Build history of the part. All positions in model axes, mm. A direction names the side the tool comes from. Coordinates: 2 decimals unless noted, no trailing zeros. Loops run counter-clockwise (first coordinate to the right, second up) from the corner with the lowest first, then second, coordinate; pieces in that order, holes last.
Item 1: Mould opens along X. For faces 6 (the face through (94.38, 0.79, -65.22)), 7 (the face through (36.611, 0.789, -8.294)), 8 (the face through (56, 1.6, -36)), 9 (the face through (19.304, 0.789, -61.17)) say: released by +X, released by -X, zero draft, split by the parting line, or undercut.
Item 2: Cut at A-A (z = -32.5). List the corners of the cut face in (x, y), and give its area (3 significant figures).
Item 3: 3-axis set-ups, long thin cutter, end or side, ignore diameter. For faces 1 (the face through (17.121, 0.789, 0.224)), 2 (the face through (84.459, 0.789, 3.984)), 3 (the face through (79.23, 0.79, -50.7)), 4 (the face through (81.82, 0.79, -5.3)), 5 (the face through (88.41, 0.79, -71.1)): which of +Z, -Z, +X, -X, +Y, -Y reach the whole face in a straight line?
Item 4: Drill centre lines: line 1 along X through (y, z) = (1, -52.5); line 2 along X through (y, z) = (0.45, 0); line 3 along Z through (x, y) = (27.5, 0.75). Where is each one in solid material? Low to high.
Item 5: Cut at D-D (z = -49.5). List the corners of the cut face in (x, y), and give its area (3 significant figures).
Item 6: Flat gauge pin, fed straight in: pin 1 (0.5 mm diameter, centred on x = 58, y = 0.5, fed in from -Z). Where does the tip first touch, or does it go through?
Item 7: Cut at B-B (x = 59). List the corners of the cut face in (y, z), and give its area (3 significant figures).
Item 8: Cut at C-C (y = 0.95). Count the separate pieces of the cut face and the enclosed holes in it, and give its area (3 significant figures).
from build123d import *

# Parameters (mm, degrees)
EXTRUDE_1_DEPTH     = 1.6
SKETCH_2_R          = 3.5
SKETCH_2_R_2        = 1.5
CUT_EXTRUDE_2_DEPTH = 120.775748848


with BuildPart() as part:
    # 草图1 → 凸台-拉伸1 (new body)
    with BuildSketch(Plane(origin=(0, 0, 0), x_dir=(1, 0, 0), z_dir=(0, 1, 0))):
        with BuildLine():
            Line((47.950455462, 53.500678068), (63.550455462, 53.500678068))
            ThreePointArc((63.550455462, 53.500678068), (64.200939835, 53.197825288), (64.387892442, 52.505078257))
            ThreePointArc((64.387892442, 52.505078257), (64.672019835, 51.714227719), (65.496953127, 51.554046536))
            ThreePointArc((65.496953127, 51.554046536), (76.012452894, 57.657876981), (83.307978073, 67.384530764))
            ThreePointArc((83.307978073, 67.384530764), (84.439034072, 68.966777391), (86.050077403, 70.056424786))
            Line((86.050077403, 70.056424786), (90.83225012, 72.174467215))
            ThreePointArc((90.83225012, 72.174467215), (91.420402092, 72.243211116), (91.944318718, 71.967240399))
            Line((91.944318718, 71.967240399), (93.014982831, 70.896576286))
            Line((93.014982831, 70.896576286), (91.559408573, 69.441002029))
            ThreePointArc((91.559408573, 69.441002029), (92.166454693, 68.916677299), (92.690779423, 68.309631179))
            Line((92.690779423, 68.309631179), (94.146353681, 69.765205436))
            Line((94.146353681, 69.765205436), (95.217017793, 68.694541323))
            ThreePointArc((95.217017793, 68.694541323), (95.49298851, 68.170624698), (95.424244609, 67.582472725))
            Line((95.424244609, 67.582472725), (93.306202181, 62.800300009))
            ThreePointArc((93.306202181, 62.800300009), (92.216554786, 61.189256677), (90.634308158, 60.058200679))
            ThreePointArc((90.634308158, 60.058200679), (79.105768954, 50.532503354), (73.491163469, 36.671683358))
            ThreePointArc((73.491163469, 36.671683358), (73.672060349, 35.948096267), (74.303399444, 35.550965423))
            ThreePointArc((74.303399444, 35.550965423), (76.850455462, 32.500678068), (74.303399444, 29.450390712))
            ThreePointArc((74.303399444, 29.450390712), (73.672060349, 29.053259868), (73.491163469, 28.329672777))
            ThreePointArc((73.491163469, 28.329672777), (79.105768724, 14.468853095), (90.634307454, 4.94315579))
            ThreePointArc((90.634307454, 4.94315579), (92.216554514, 3.812099737), (93.306202181, 2.201056127))
            Line((93.306202181, 2.201056127), (95.424244609, -2.58111659))
            ThreePointArc((95.424244609, -2.58111659), (95.49298851, -3.169268563), (95.217017793, -3.693185188))
            Line((95.217017793, -3.693185188), (94.146353681, -4.763849301))
            Line((94.146353681, -4.763849301), (92.690779423, -3.308275044))
            ThreePointArc((92.690779423, -3.308275044), (92.166454693, -3.915321163), (91.559408573, -4.439645893))
            Line((91.559408573, -4.439645893), (93.014982831, -5.895220151))
            Line((93.014982831, -5.895220151), (91.944318718, -6.965884264))
            ThreePointArc((91.944318718, -6.965884264), (91.420402092, -7.24185498), (90.83225012, -7.173111079))
            Line((90.83225012, -7.173111079), (86.050077403, -5.055068651))
            ThreePointArc((86.050077403, -5.055068651), (84.439034072, -3.965421256), (83.307978073, -2.383174628))
            ThreePointArc((83.307978073, -2.383174628), (75.037180063, 8.17430315), (63.037239962, 14.163282556))
            ThreePointArc((63.037239962, 14.163282556), (61.901454693, 13.989537546), (61.221822682, 13.063094977))
            ThreePointArc((61.221822682, 13.063094977), (60.867876271, 12.514045024), (60.250455462, 12.300678068))
            Line((60.250455462, 12.300678068), (51.250455462, 12.300678068))
            ThreePointArc((51.250455462, 12.300678068), (50.633034654, 12.514045024), (50.279088243, 13.063094977))
            ThreePointArc((50.279088243, 13.063094977), (49.599456231, 13.989537546), (48.463670963, 14.163282556))
            ThreePointArc((48.463670963, 14.163282556), (36.463730861, 8.17430315), (28.192932851, -2.383174628))
            ThreePointArc((28.192932851, -2.383174628), (27.061876853, -3.965421256), (25.450833521, -5.055068651))
            Line((25.450833521, -5.055068651), (20.668660805, -7.173111079))
            ThreePointArc((20.668660805, -7.173111079), (20.080508832, -7.24185498), (19.556592206, -6.965884264))
            Line((19.556592206, -6.965884264), (18.485928094, -5.895220151))
            Line((18.485928094, -5.895220151), (19.941502351, -4.439645893))
            ThreePointArc((19.941502351, -4.439645893), (19.334456231, -3.915321163), (18.810131501, -3.308275044))
            Line((18.810131501, -3.308275044), (17.354557244, -4.763849301))
            Line((17.354557244, -4.763849301), (16.283893131, -3.693185188))
            ThreePointArc((16.283893131, -3.693185188), (16.007922414, -3.169268563), (16.076666315, -2.58111659))
            Line((16.076666315, -2.58111659), (18.194708744, 2.201056127))
            ThreePointArc((18.194708744, 2.201056127), (19.28435641, 3.812099737), (20.86660347, 4.94315579))
            ThreePointArc((20.86660347, 4.94315579), (32.395142201, 14.468853095), (38.009747455, 28.329672777))
            ThreePointArc((38.009747455, 28.329672777), (37.828850575, 29.053259868), (37.19751148, 29.450390712))
            ThreePointArc((37.19751148, 29.450390712), (34.650455462, 32.500678068), (37.19751148, 35.550965423))
            ThreePointArc((37.19751148, 35.550965423), (37.828850575, 35.948096267), (38.009747455, 36.671683358))
            ThreePointArc((38.009747455, 36.671683358), (32.39514197, 50.532503354), (20.866602766, 60.058200679))
            ThreePointArc((20.866602766, 60.058200679), (19.284356139, 61.189256677), (18.194708744, 62.800300009))
            Line((18.194708744, 62.800300009), (16.076666315, 67.582472725))
            ThreePointArc((16.076666315, 67.582472725), (16.007922414, 68.170624698), (16.283893131, 68.694541323))
            Line((16.283893131, 68.694541323), (17.354557244, 69.765205436))
            Line((17.354557244, 69.765205436), (18.810131501, 68.309631179))
            ThreePointArc((18.810131501, 68.309631179), (19.334456231, 68.916677299), (19.941502351, 69.441002029))
            Line((19.941502351, 69.441002029), (18.485928094, 70.896576286))
            Line((18.485928094, 70.896576286), (19.556592206, 71.967240399))
            ThreePointArc((19.556592206, 71.967240399), (20.080508832, 72.243211116), (20.668660805, 72.174467215))
            Line((20.668660805, 72.174467215), (25.450833521, 70.056424786))
            ThreePointArc((25.450833521, 70.056424786), (27.061876853, 68.966777391), (28.192932851, 67.384530764))
            ThreePointArc((28.192932851, 67.384530764), (35.488458031, 57.657876981), (46.003957797, 51.554046536))
            ThreePointArc((46.003957797, 51.554046536), (46.82889109, 51.714227719), (47.113018482, 52.505078257))
            ThreePointArc((47.113018482, 52.505078257), (47.299971089, 53.197825288), (47.950455462, 53.500678068))
        make_face()
    extrude(amount=EXTRUDE_1_DEPTH)

    # 草图2 → 切除-拉伸2 (cut, through all)
    with BuildSketch(Plane(origin=(0, 0, 0), x_dir=(1, 0, 0), z_dir=(0, 1, 0))):
        with Locations(Location((88.277367397, -0.026233867, 0), (0, 0, 270))):
            Circle(SKETCH_2_R)
        with Locations(Location((88.277367397, 65.027590002, 0), (0, 0, 270))):
            Circle(SKETCH_2_R)
        with Locations(Location((23.223543528, -0.026233867, 0), (0, 0, 270))):
            Circle(SKETCH_2_R)
        with Locations(Location((23.223543528, 65.027590002, 0), (0, 0, 270))):
            Circle(SKETCH_2_R)
        with Locations(Location((37.750455462, 32.500678068, 0), (0, 0, 270))):
            Circle(SKETCH_2_R_2)
        with Locations(Location((73.750455462, 32.500678068, 0), (0, 0, 270))):
            Circle(SKETCH_2_R_2)
        with BuildLine():
            Line((84.3882801, 4.994224279), (81.559852975, 7.822651404))
            ThreePointArc((81.559852975, 7.822651404), (80.428482126, 7.822651404), (80.428482126, 6.691280554))
            Line((80.428482126, 6.691280554), (83.25690925, 3.86285343))
            ThreePointArc((83.25690925, 3.86285343), (84.3882801, 3.86285343), (84.3882801, 4.994224279))
        make_face()
        with BuildLine():
            Line((27.112630824, 60.007131856), (29.941057949, 57.178704731))
            ThreePointArc((29.941057949, 57.178704731), (31.072428799, 57.178704731), (31.072428799, 58.310075581))
            Line((31.072428799, 58.310075581), (28.244001674, 61.138502706))
            ThreePointArc((28.244001674, 61.138502706), (27.112630824, 61.138502706), (27.112630824, 60.007131856))
        make_face()
        with BuildLine():
            Line((27.112630824, 4.994224279), (29.941057949, 7.822651404))
            ThreePointArc((29.941057949, 7.822651404), (31.072428799, 7.822651404), (31.072428799, 6.691280554))
            Line((31.072428799, 6.691280554), (28.244001674, 3.86285343))
            ThreePointArc((28.244001674, 3.86285343), (27.112630824, 3.86285343), (27.112630824, 4.994224279))
        make_face()
        with BuildLine():
            Line((84.3882801, 60.007131856), (81.559852975, 57.178704731))
            ThreePointArc((81.559852975, 57.178704731), (80.428482126, 57.178704731), (80.428482126, 58.310075581))
            Line((80.428482126, 58.310075581), (83.25690925, 61.138502706))
            ThreePointArc((83.25690925, 61.138502706), (84.3882801, 61.138502706), (84.3882801, 60.007131856))
        make_face()
    extrude(amount=CUT_EXTRUDE_2_DEPTH, mode=Mode.SUBTRACT)


solid = part.part
Filled sheet:
1. face 6: released by +X
1. face 7: undercut
1. face 8: zero draft
1. face 9: released by -X
2. outline: (34.65, 0) - (36.25, 0) - (36.25, 1.6) - (34.65, 1.6) - close; (39.25, 0) - (72.25, 0) - (72.25, 1.6) - (39.25, 1.6) - close; (75.25, 0) - (76.85, 0) - (76.85, 1.6) - (75.25, 1.6) - close
2. area: 57.9 mm2
3. face 1: -X, +Y, -Y
3. face 2: +Z, +Y, -Y
3. face 3: +X, +Y, -Y
3. face 4: +Y, -Y
3. face 5: -Z, +Y, -Y
4. line 1: x = 30.82 to 43.55, 47.11 to 64.39, 67.95 to 80.68
4. line 2: x = 17.22 to 19.72, 26.72 to 29.46, 82.05 to 84.78, 91.78 to 94.28
4. line 3: z = -68.49 to -61.35, -59.62 to -55.78, -9.22 to -5.38, -3.65 to 3.48
5. outline: (33.12, 0) - (78.38, 0) - (78.38, 1.6) - (33.12, 1.6) - close
5. area: 72.4 mm2
6. pin 1: stops at z = -53.5
7. outline: (0, -53.5) - (1.6, -53.5) - (1.6, -12.3) - (0, -12.3) - close
7. area: 65.9 mm2
8. separate pieces: 1
8. enclosed holes: 10
8. area: 2,250 mm2
